For this review, take the finished solid that the model builds, in its own axes (mm). A direction names the side the tool comes from. Give positions to 0.01 mm unless a question says otherwise; leave off trailing zeros. Loops run counter-clockwise (first coordinate to the right, second up) from the corner with the lowest first, then second, coordinate; pieces in that order, holes last. Notation, with made-up numbers: (71.5, -29) -> (88.5, -29) arc R7 cw to (88.5, -16) -> close; hole circle Ø8 at (64.25, 28.5). An arc over 180 degrees is marked (long way). One line per question, with ' | ' between items. Start each with the question number.
(1) Insertion check: P1, Ø2.5, axis at y = -2, z = 5.5, coming from the -X side; P2, Ø3, axis at y = -63.5, z = -49, coming from the +X side; P3, Ø5, axis at x = 69, y = 9, coming from the -Z side; P4, Ø9.5, axis at x = 118.5, z = 6.5, coming from the -Y side. Each pin has a flat end and moves straight along its axis. Give the tip position at first contact, or say it passes through.
(2) Tool access review of faces 1 (the flat face through (105, -4.906, 6)), 2 (the cylindrical face through (297.117, 24.03, 76.306)), 3 (the flat face through (295, -16, 1)): name each direction out of +Z, -Z, +X, -X, +Y, -Y from which nothing blocks a thin tool from reaching the whole face with its end or side.
(3) Draft analysis for pull direction Y (two halves, no side actions). For faces 4 (the cylindrical face through (304.86, 0.66, -14.985)), 5 (the flat face through (0, 0, 0)), 6 (the cylindrical face through (138.448, 0.55, -12.488)), state which applies: +Y half, -Y half, draft (parallel to the pull), parting line (faces both ways), or undercut.
(4) Wall thickness on probe 1 along Y at (x, z) = (296, 0); probe 2 along X at (y, z) = (-65.5, 38.5); probe 3 along X at (y, z) = (-57, -10): over which ranges is each line inside the solid? List them lowest first.
(5) Consider section A-A (x = 228). Write out the cut boundary in (y, z), and give its area (3 significant figures).
from build123d import *

# Parameters (mm, degrees)
F2_W     = 70
F2_H     = 8
F3_DEPTH = 12.501
F4_R     = 5
F5_R     = 5


with BuildPart() as f1:
    # F0 (on Front) → F1 (revolve)
    with BuildSketch(Plane.XZ):
        Polygon((0, 12.5), (0, 0), (295, 0), (315, 0), (315, 15), (295, 15), (295, 75), (300, 75), (300, 80), (290, 80), (280, 12.5), align=None)
    revolve(axis=Axis((147.5, 0, 0), (-1, 0, 0)))

    # F2 (on Top) → F3 (cut, through all)
    with BuildSketch(Plane.XY):
        with Locations((105, -0.9058431759)):
            Rectangle(F2_W, F2_H)
    extrude(amount=F3_DEPTH, mode=Mode.SUBTRACT)

    # F4
    f4_edges = [f1.edges().sort_by_distance(p)[0] for p in [
        (290, 0, -80),
        (280, 0, -12.5),
    ]]
    fillet(f4_edges, radius=F4_R)

    # F5
    f5_edges = [f1.edges().sort_by_distance(p)[0] for p in [
        (0, 0, -12.5),
    ]]
    fillet(f5_edges, radius=F5_R)


solid = f1.part
A:
1) P1: stops at x = 0 | P2: stops at x = 300 | P3: stops at z = -10.68 | P4: stops at y = -12.38
2) face 1: +Z | face 2: +X, -X | face 3: +X
3) face 4: undercut | face 5: draft | face 6: parting line
4) probe 1: y = -80 to -75, -15 to 15, 75 to 80 | probe 2: x = 289.41 to 300 | probe 3: x = 286.72 to 295
5) outline: circle Ø25 at (0, 0) | area: 491 mm^2
